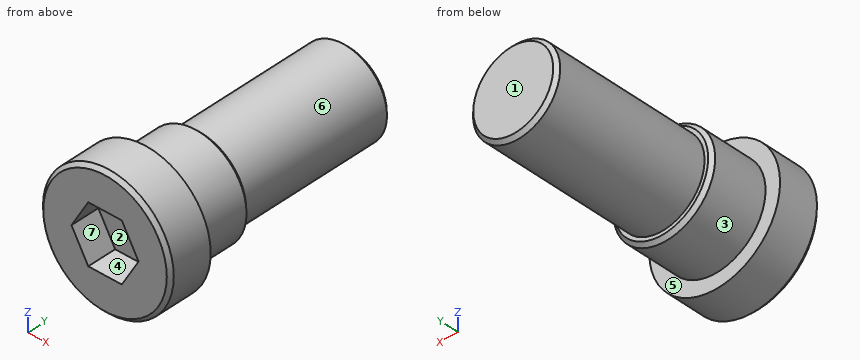
from build123d import *

# Parameters (mm, degrees)
CUT_EXTRUDE1_DEPTH = 1
CHAMFER1_SIZE      = 0.125


with BuildPart() as part:
    # Sketch1 → Revolve1 (revolve)
    with BuildSketch(Plane.XY):
        Polygon((0, 0), (0, 9), (1.5, 9), (1.5, 3.5), (1.75, 3.5), (1.75, 1.5), (2.25, 1.5), (2.25, 0), align=None)
    revolve(axis=Axis((0, 0, 0), (0, -1, 0)))

    # Sketch2 → Cut-Extrude1 (cut)
    with BuildSketch(Plane.XZ):
        Polygon((1.154700538, 0), (0.577350269, 1), (-0.577350269, 1), (-1.154700538, 0), (-0.577350269, -1), (0.577350269, -1), align=None)
    extrude(amount=-CUT_EXTRUDE1_DEPTH, mode=Mode.SUBTRACT)

    # Chamfer1
    chamfer1_edges = [part.edges().sort_by_distance(p)[0] for p in [
        (-2.25, 0, 0),
        (-1.75, 3.5, 0),
        (-1.5, 9, 0),
    ]]
    chamfer(chamfer1_edges, length=CHAMFER1_SIZE)


solid = part.part
Work out the finished part from the listing and answer in its coordinate system (mm). Face numbers are marked on the shaded views. A direction names the side the tool comes from. Coordinates: 2 decimals unless noted, no trailing zeros. Write each loop counter-clockwise with the first axis right and the second up, starting at its lowest first coordinate (ties: lowest second). Pieces come first, ordered by that corner, then holes.
1. The part is cut by section D-D, the plane y = 5.75. Write down the section's boundary in (x, z).
Results list:
outline: circle Ø3 at (0, 0)
2. For the marked faces 1, 2 and 3, determine the directions among +Z, -Z, +X, -X, +Y, -Y from which every point of the face is accessible in a straight line to the end or side of a thin tool.
Results list:
face 1: +Z, -Z, +X, -X, +Y
face 2: -Y
face 3: +Y
3. Flat-ended cylindrical pins translate along their axes: pin 1 (1 mm diameter, centred on x = 0, y = 8, fed in from -Z); pin 2 (0.6 mm diameter, centred on x = 0, z = 0.5, fed in from -Y). Find the tip coordinate at first contact, or state that the pin passes through.
Results list:
pin 1: stops at z = -1.5
pin 2: stops at y = 1
4. The part is cut by section C-C, the plane y = 2.75. Write down the section's boundary in (x, z), and give its area (3 significant figures).
Results list:
outline: circle Ø3.5 at (0, 0)
area: 9.62 mm2
5. The part is cut by section A-A, the plane y = 0.5. Write down the section's boundary in (x, z).
Results list:
outline: circle Ø4.5 at (0, 0); hole (-1.15, 0) - (-0.58, -1) - (0.58, -1) - (1.15, 0) - (0.58, 1) - (-0.58, 1) - close
6. Consider line 1 along Y through (x, z) = (-1.15, 1.45); line 2 along Z through (x, y) = (-0.5, 0.75); line 3 along Y through (x, z) = (0.4, -0.4). Determine where each line is inside the solid, lowest interval first.
Results list:
line 1: y = 0 to 1.5
line 2: z = -2.19 to -1, 1 to 2.19
line 3: y = 1 to 9
7. The part is cut by section B-B, the plane x = 0. Write down the section's boundary in (y, z) (3 decimals).
Results list:
outline: (0, -2.125) - (0.125, -2.25) - (1.5, -2.25) - (1.5, -1.75) - (3.375, -1.75) - (3.5, -1.625) - (3.5, -1.5) - (8.875, -1.5) - (9, -1.375) - (9, 1.375) - (8.875, 1.5) - (3.5, 1.5) - (3.5, 1.625) - (3.375, 1.75) - (1.5, 1.75) - (1.5, 2.25) - (0.125, 2.25) - (0, 2.125) - (0, 1) - (1, 1) - (1, -1) - (0, -1) - close
8. For a pull along X with two mould halves and no side action, classify the marked faces 4, 5, 6 and 7 as +X half, -X half, draft (parallel to the pull), parting line (faces both ways), or undercut.
Results list:
face 4: undercut
face 5: draft
face 6: parting line
face 7: undercut
